from build123d import *

# Parameters (mm, degrees)
SKETCH1_W           = 15
SKETCH1_H           = 20
BOSS_EXTRUDE1_DEPTH = 30
CUT_EXTRUDE1_REACH  = 37
SKETCH4_W           = 6
SKETCH4_H           = 6
CUT_EXTRUDE4_DEPTH  = 25
CUT_EXTRUDE2_REACH  = 34.5
SKETCH3_R           = 1.1


with BuildPart() as part:
    # Sketch1 → Boss-Extrude1 (new body)
    with BuildSketch(Plane(origin=(0, 0, 0), x_dir=(1, 0, 0), z_dir=(0, 1, 0))):
        Rectangle(SKETCH1_W, SKETCH1_H)
    extrude(amount=BOSS_EXTRUDE1_DEPTH)

    # Sketch2 → Cut-Extrude1 (cut, up to next)
    with BuildSketch(Plane(origin=(7.5, 0, 0), x_dir=(0, 0, -1), z_dir=(1, 0, 0)), mode=Mode.PRIVATE) as cut_extrude1_sk1:
        with BuildLine():
            Line((-10, 3), (-10, 27))
            ThreePointArc((-10, 27), (2, 15), (-10, 3))
        make_face()
    cut_extrude1_tool1 = extrude(cut_extrude1_sk1.sketch, amount=-CUT_EXTRUDE1_REACH, mode=Mode.PRIVATE) & part.part
    add(cut_extrude1_tool1.solids().sort_by_distance((7.5, 15, 4.907042))[0], mode=Mode.SUBTRACT)

    # Sketch4 → Cut-Extrude4 (cut)
    with BuildSketch(Plane(origin=(0, 30, 0), x_dir=(1, 0, 0), z_dir=(0, 1, 0))):
        with Locations((0, 7)):
            Rectangle(SKETCH4_W, SKETCH4_H)
    extrude(amount=-CUT_EXTRUDE4_DEPTH, mode=Mode.SUBTRACT)

    # Sketch3 → Cut-Extrude2 (cut, up to next)
    with BuildSketch(Plane(origin=(0, 30, 0), x_dir=(1, 0, 0), z_dir=(0, 1, 0)), mode=Mode.PRIVATE) as cut_extrude2_sk1:
        with Locations(Location((0, 7, 0), (0, 0, 270))):
            Circle(SKETCH3_R)
    cut_extrude2_tool1 = extrude(cut_extrude2_sk1.sketch, amount=-CUT_EXTRUDE2_REACH, mode=Mode.PRIVATE) & part.part
    add(cut_extrude2_tool1.solids().sort_by_distance((0, 30, -7))[0], mode=Mode.SUBTRACT)


solid = part.part
Design review of the part built by this model. Coordinates are the model's own, in mm. A direction names the side the tool comes from. Round coordinates to 2 decimals unless told otherwise and drop trailing zeros. Write each loop counter-clockwise with the first axis right and the second up, starting at its lowest first coordinate (ties: lowest second). Pieces come first, ordered by that corner, then holes. Notation, with made-up numbers: (52.5, 16) - (70.5, 16) arc R15 ccw to (70.5, 33) - close; hole circle Ø9 at (55.5, 18). An arc over 180 degrees is marked (long way). Return JSON: item names as keys, results as strings. Group by question number.
Item 1: For probe 1 along X at (y, z) = (3.1, -7); probe 2 along Y at (x, z) = (3.25, 7.5); probe 3 along Y at (x, z) = (-3.75, 5.25), list the stretches that pass through material, from the lowest coordinate up. Write a range as [from, to].
Item 2: We need section D-D on z = 3. Write out the cut boundary in (x, y).
Item 3: We need section B-B on y = 15. Write out the cut boundary in (x, z), and give its area (3 significant figures).
Item 4: The part is to be moulded in two halves that separate along X. For faces 3 (the face through (-3, 18, -7)), 4 (the face through (7.5, 15, -4)), 5 (the face through (-7.5, 15, -4)), 6 (the face through (0, 30, 0)), say which applies: pulls with the +X half, pulls with the -X half, needs draft (parallel to the pull), parting line crosses it, or undercut.
Item 5: Machinability: for faces 1 (the face through (0, 1, 10)), 2 (the face through (3, 18, -7)), which of the approach directions +Z, -Z, +X, -X, +Y, -Y give a long, thin tool a straight path to every point of the face, cutting with its end or side? Answer none if there is none.
Item 6: We need section A-A on z = -7. Write out the cut boundary in (x, y).
Item 7: Insertion check: P1, Ø6.5, axis at x = -0.5, z = -6.5, coming from the +Y side; P2, Ø3, axis at x = 0, z = -7, coming from the +Y side; P3, Ø5, axis at x = 6, y = 19, coming from the +Z side. Each pin has a flat end and moves straight along its axis. Give the tip position at first contact, or say it passes through.
Item 8: We need section C-C on x = 3.5. Write out the cut boundary in (y, z).
Model answer:
{
 "1": {"probe 1": "x = [-7.5, -1.1], [1.1, 7.5]", "probe 2": "y = [0, 3.26], [26.74, 30]", "probe 3": "y = [0, 3.98], [26.02, 30]"},
 "2": {"outline": "(-7.5, 0) - (7.5, 0) - (7.5, 5.25) - (-7.5, 5.25) - close; (-7.5, 24.75) - (7.5, 24.75) - (7.5, 30) - (-7.5, 30) - close"},
 "3": {"outline": "(-7.5, -10) - (-3, -10) - (-3, -4) - (3, -4) - (3, -10) - (7.5, -10) - (7.5, -2) - (-7.5, -2) - close", "area": "84.0 mm²"},
 "4": {"face 3": "undercut", "face 4": "pulls with the +X half", "face 5": "pulls with the -X half", "face 6": "needs draft"},
 "5": {"face 1": "+Z, +X, -X, +Y, -Y", "face 2": "-Z, +Y"},
 "6": {"outline": "(-7.5, 0) - (-1.1, 0) - (-1.1, 5) - (-3, 5) - (-3, 30) - (-7.5, 30) - close; (1.1, 0) - (7.5, 0) - (7.5, 30) - (3, 30) - (3, 5) - (1.1, 5) - close"},
 "7": {"P1": "stops at y = 30", "P2": "stops at y = 5", "P3": "stops at z = -0.09"},
 "8": {"outline": "(0, -10) - (30, -10) - (30, 10) - (27, 10) arc R12 cw to (3, 10) - (0, 10) - close"}
}
